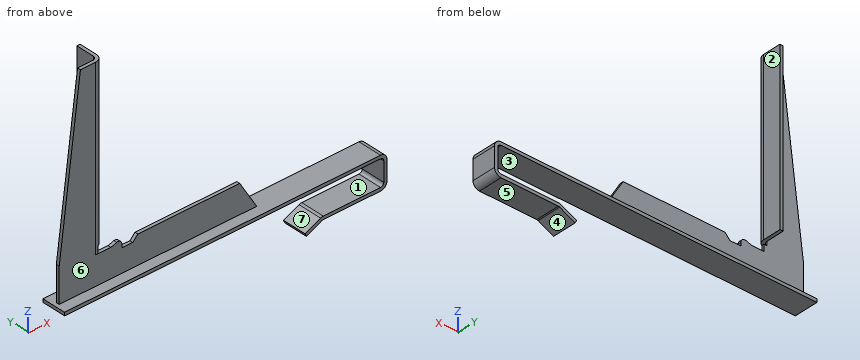
from build123d import *

# Parameters (mm, degrees)
F1_DEPTH    = 15
F3_DEPTH    = 2
F4_W        = 4
F4_H        = 28
F5_DEPTH    = 206.7509774754
F6_T1_DEPTH = 206.7509774754
F7_T4_DEPTH = 251.7509774754


# Not quite as in the source:
# - a fillet or chamfer that OpenCascade refuses, or shapes differently, is made with other operations: its cross-section is extruded or revolved along the edge and cut away or added


with BuildPart() as f1:
    # F0 (on Front) → F1 (new body, symmetric)
    with BuildSketch(Plane.XZ):
        with BuildLine():
            Line((180.6789295077, 32.8460444401), (-211.3210704923, 32.8460444401))
            Line((-211.3210704923, 32.8460444401), (-211.3210704923, 28.8460444401))
            Line((-211.3210704923, 28.8460444401), (180.6789295077, 28.8460444401))
            ThreePointArc((180.6789295077, 28.8460444401), (183.5073566325, 27.6744715648), (184.6789295077, 24.8460444401))
            Line((184.6789295077, 24.8460444401), (184.6789295077, 0.8460444401))
            ThreePointArc((184.6789295077, 0.8460444401), (183.5073566325, -1.9823826847), (180.6789295077, -3.1539555599))
            Line((180.6789295077, -3.1539555599), (109.5657081583, -3.1539555599))
            ThreePointArc((109.5657081583, -3.1539555599), (107.8341912468, -3.343587503), (106.1847620644, -3.9034932637))
            Line((106.1847620644, -3.9034932637), (86.9884564608, -12.8548775749))
            Line((86.9884564608, -12.8548775749), (88.6789295077, -16.480108723))
            Line((88.6789295077, -16.480108723), (107.8752351113, -7.5287244118))
            ThreePointArc((107.8752351113, -7.5287244118), (108.6999497026, -7.2487715315), (109.5657081583, -7.1539555599))
            Line((109.5657081583, -7.1539555599), (180.6789295077, -7.1539555599))
            ThreePointArc((180.6789295077, -7.1539555599), (186.3357837572, -4.8108098094), (188.6789295077, 0.8460444401))
            Line((188.6789295077, 0.8460444401), (188.6789295077, 24.8460444401))
            ThreePointArc((188.6789295077, 24.8460444401), (186.3357837572, 30.5028986895), (180.6789295077, 32.8460444401))
        make_face()
    extrude(amount=F1_DEPTH, both=True)

    # F2 (on Front) → F3 (join, symmetric)
    with BuildSketch(Plane.XZ):
        with BuildLine():
            Line((-206.3210704923, 75.6694748998), (-206.3210704923, 32.8460444401))
            Line((-206.3210704923, 32.8460444401), (38.6789295077, 32.8460444401))
            Line((38.6789295077, 32.8460444401), (17.569155556, 67.8460444401))
            Line((17.569155556, 67.8460444401), (-108.8612323146, 67.8460444401))
            Line((-108.8612323146, 67.8460444401), (-115.0114574584, 61.1853342652))
            Line((-115.0114574584, 61.1853342652), (-128.5433099752, 61.1853342652))
            Line((-128.5433099752, 61.1853342652), (-128.5433099752, 65.3464212941))
            ThreePointArc((-128.5433099752, 65.3464212941), (-130.579832864, 69.3735546928), (-135.0304313397, 70.1201483545))
            Line((-135.0304313397, 70.1201483545), (-142.3304080963, 67.8460444401))
            Line((-142.3304080963, 67.8460444401), (-157.2653103035, 67.8460444401))
            Line((-157.2653103035, 67.8460444401), (-157.2653103035, 76.0950669646))
            Line((-157.2653103035, 76.0950669646), (-152.0575187367, 76.0950669646))
            Line((-152.0575187367, 76.0950669646), (-152.0575187367, 282.8460444401))
            Line((-152.0575187367, 282.8460444401), (-180.0575187367, 282.8460444401))
            Line((-180.0575187367, 282.8460444401), (-206.3210704923, 75.6694748998))
        make_face()
    extrude(amount=F3_DEPTH, both=True)

    # F4 (on face) → F5 (join, through all)
    with BuildSketch(Plane.XY.offset(282.8460444401)):
        with Locations((-154.0575187367, 16)):
            Rectangle(F4_W, F4_H)
    extrude(amount=-F5_DEPTH)

    # F6: fillet of radius 5 on 1 edges, made by hand

    # F6_s2 → F6_t1 (join)
    with BuildSketch(Plane.XY.offset(76.0950669646)):
        with BuildLine():
            ThreePointArc((-161.0575187367, 2), (-157.5219848308, 3.4644660941), (-156.0575187367, 7))
            Line((-156.0575187367, 7), (-156.0575187367, 2))
            Line((-156.0575187367, 2), (-161.0575187367, 2))
        make_face()
    extrude(amount=F6_T1_DEPTH)

    # F7: fillet of radius 9 on 1 edges, made by hand


with BuildPart() as f7_tool2:
    # F7_s3 → F7_t4 (new body)
    with BuildSketch(Plane.XY.offset(53.5950669646)):
        with BuildLine():
            ThreePointArc((-161.0575187367, -2), (-154.6935577061, 0.6360389693), (-152.0575187367, 7))
            Line((-152.0575187367, 7), (-152.0575187367, -2))
            Line((-152.0575187367, -2), (-161.0575187367, -2))
        make_face()
    extrude(amount=F7_T4_DEPTH)

    split(bisect_by=Plane.XY.offset(67.8460444401), keep=Keep.TOP)


with BuildPart() as f1_1:
    add(f1.part)

    # F7_t1: cut F7_tool2
    add(f7_tool2.part, mode=Mode.SUBTRACT)


solid = f1_1.part
Design review of the part built by this model. Coordinates are the model's own, in mm. Face numbers are marked on the shaded views. A direction names the side the tool comes from. Round coordinates to 2 decimals unless told otherwise and drop trailing zeros. Order: outer loops, then holes, each group sorted by start corner. A loop starts at its lowest first (then second) coordinate and runs counter-clockwise, first axis right, second up.
1) Consider section B-B (z = 193.5). State the section outline as (x, y) points, plus the area to 3 significant figures.
The answers:
outline: (-191.38, -2) - (-161.06, -2) arc R9 ccw to (-152.06, 7) - (-152.06, 30) - (-156.06, 30) - (-156.06, 7) arc R5 cw to (-161.06, 2) - (-191.38, 2) - close
area: 257 mm2
2) Clearance check with flat-ended pins moving along their axes: pin 1 Ø1.5 at (x, y) = (1, 10.5) entering from -Z; pin 2 Ø12 at (y, z) = (-6.5, 8) entering from -X; pin 3 Ø4.5 at (x, y) = (-123.5, 0.5) entering from +Z; pin 4 Ø5 at (y, z) = (-5, 105.5) entering from +X. State where each tip first meets the part, or that it passes through.
The answers:
pin 1: stops at z = 28.85
pin 2: stops at x = 184.68
pin 3: stops at z = 61.19
pin 4: passes through
3) For L1, parallel to X at y = 18, z = 106.5; L2, parallel to Z at x = -144.5, y = -1; L3, parallel to Z at x = -78, y = -6.5, list the stretches that pass through material, from the lowest coordinate up.
The answers:
L1: x = -156.06 to -152.06
L2: z = 28.85 to 67.85
L3: z = 28.85 to 32.85
4) Consider section C-C (y = 20). State the section outline as (x, z) points, plus the area to 3 significant figures.
The answers:
outline: (-156.06, 76.1) - (-152.06, 76.1) - (-152.06, 282.85) - (-156.06, 282.85) - close
area: 827 mm2
5) Draft analysis for pull direction Z (two halves, no side actions). For the marked faces 1, 2, 3 and 4, state which applies: released by +Z, released by -Z, zero draft, split by the parting line, or undercut.
The answers:
face 1: undercut
face 2: zero draft
face 3: undercut
face 4: released by -Z
6) Machinability: for the marked faces 5, 6 and 7, which of the approach directions +Z, -Z, +X, -X, +Y, -Y give a long, thin tool a straight path to every point of the face, cutting with its end or side? Answer none if there is none.
The answers:
face 5: -Z, +X, +Y, -Y
face 6: +Z, +X, -X, -Y
face 7: -X, +Y, -Y
7) Consider section D-D (z = 5). State the section outline as (x, y) points, plus the area to 3 significant figures.
The answers:
outline: (184.68, -15) - (188.68, -15) - (188.68, 15) - (184.68, 15) - close
area: 120 mm2
8) Consider section A-A (x = -171). State the section outline as (y, z) points.
The answers:
outline: (-15, 28.85) - (15, 28.85) - (15, 32.85) - (2, 32.85) - (2, 282.85) - (-2, 282.85) - (-2, 32.85) - (-15, 32.85) - close
